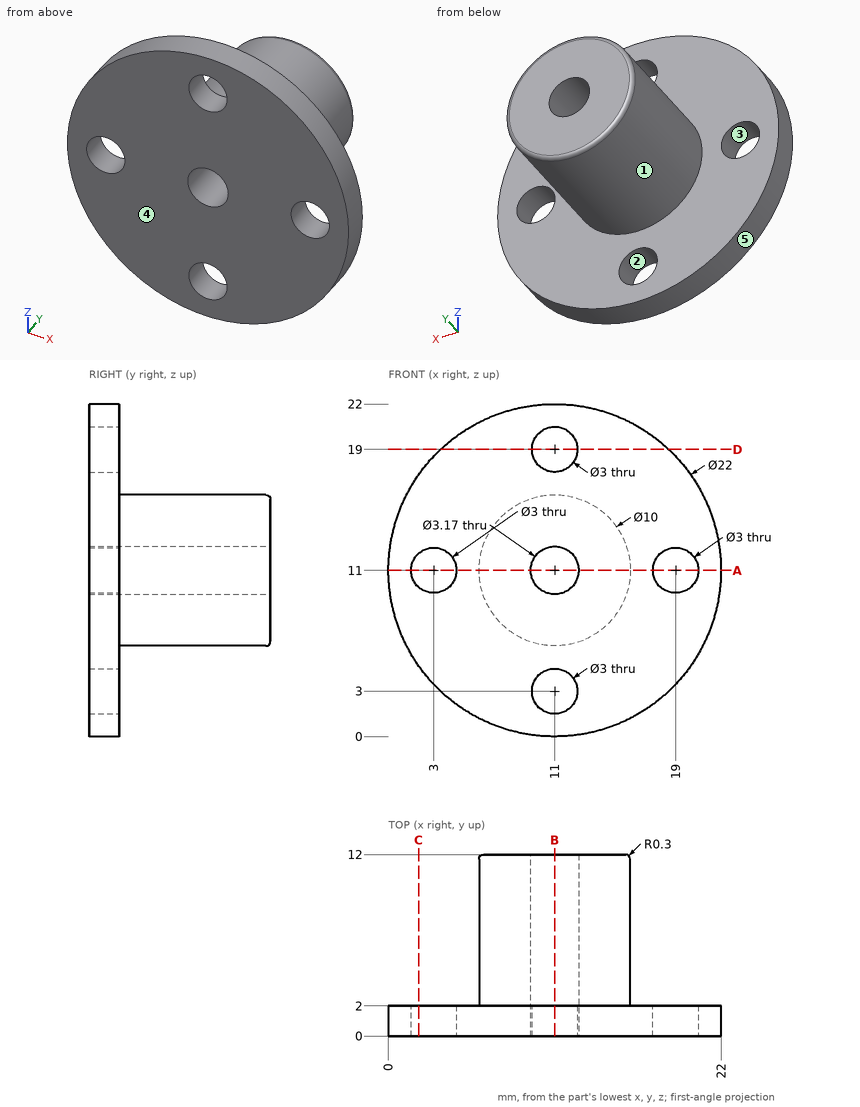
For this review, use the dimensioned drawing (mm, ordinates from the lowest corner) and the shaded views. A direction names the side the tool comes from. Give positions to 0.01 mm unless a question says otherwise; leave off trailing zeros. Loops run counter-clockwise (first coordinate to the right, second up) from the corner with the lowest first, then second, coordinate; pieces in that order, holes last.
Item 1: Take a section at B-B, the plane x = 11. State the section outline as (y, z) points (3 decimals), and give its area (3 significant figures).
Item 2: Draft analysis for pull direction Z (two halves, no side actions). For the marked faces 3, 4 and 5, state which applies: +Z half, -Z half, draft (parallel to the pull), parting line (faces both ways), or undercut.
Item 3: Tool access review of the marked faces 1 and 2: name each direction out of +Z, -Z, +X, -X, +Y, -Y from which nothing blocks a thin tool from reaching the whole face with its end or side.
Item 4: Insertion check: pin 1 (4 mm diameter, centred on x = 11, z = 19, fed in from +Y); pin 2 (2 mm diameter, centred on y = 8, z = 9, fed in from -X); pin 3 (6 mm diameter, centred on y = 9, z = 11, fed in from -X). Each pin has a flat end and moves straight along its axis. Give the tip position at first contact, or say it passes through.
Item 5: Take a section at A-A, the plane z = 11. State the section outline as (x, y) points (3 decimals).
Item 6: Take a section at C-C, the plane x = 2. State the section outline as (y, z) points.
Item 7: For line 1 along Z through (x, y) = (11, 0.8) (3 decimals); line 2 along X through (y, z) = (3.25, 11) (3 decimals), list the stretches that pass through material, from the lowest coordinate up.
Item 8: Take a section at D-D, the plane z = 19. State the section outline as (x, y) points, and give its area (3 significant figures).
Calculated:
1. outline: (0, 0) - (2, 0) - (2, 1.5) - (0, 1.5) - close; (0, 4.5) - (2, 4.5) - (2, 6) - (11.7, 6) arc R0.3 ccw to (12, 6.3) - (12, 9.415) - (0, 9.415) - close; (0, 12.585) - (12, 12.585) - (12, 15.7) arc R0.3 ccw to (11.7, 16) - (2, 16) - (2, 17.5) - (0, 17.5) - close; (0, 20.5) - (2, 20.5) - (2, 22) - (0, 22) - close
1. area: 93.9 mm2
2. face 3: undercut
2. face 4: draft
2. face 5: parting line
3. face 1: +Y
3. face 2: +Y, -Y
4. pin 1: stops at y = 2
4. pin 2: stops at x = 6.1
4. pin 3: stops at x = 6
5. outline: (0, 0) - (1.5, 0) - (1.5, 2) - (0, 2) - close; (4.5, 0) - (9.415, 0) - (9.415, 12) - (6.3, 12) arc R0.3 ccw to (6, 11.7) - (6, 2) - (4.5, 2) - close; (12.585, 0) - (17.5, 0) - (17.5, 2) - (16, 2) - (16, 11.7) arc R0.3 ccw to (15.7, 12) - (12.585, 12) - close; (20.5, 0) - (22, 0) - (22, 2) - (20.5, 2) - close
6. outline: (0, 4.68) - (2, 4.68) - (2, 9.88) - (0, 9.88) - close; (0, 12.12) - (2, 12.12) - (2, 17.32) - (0, 17.32) - close
7. line 1: z = 0 to 1.5, 4.5 to 9.415, 12.585 to 17.5, 20.5 to 22
7. line 2: x = 6 to 9.415, 12.585 to 16
8. outline: (3.45, 0) - (9.5, 0) - (9.5, 2) - (3.45, 2) - close; (12.5, 0) - (18.55, 0) - (18.55, 2) - (12.5, 2) - close
8. area: 24.2 mm2
